Check sheet for the drawn part. Datum: minimum x, y, z corner. Units: mm. Give positions to 0.01 mm unless a question says otherwise; leave off trailing zeros. Order: outer loops, then holes, each group sorted by start corner. A loop starts at its lowest first (then second) coordinate and runs counter-clockwise, first axis right, second up. Notation, with made-up numbers: (72.5, 5) - (120.5, 5) arc R21 ccw to (120.5, 17) - close; hole circle Ø5 at (19, 76.25). An arc over 180 degrees is marked (long way). Answer as a JSON object with one key per item and string values. Group by question number.
(1) Depth check by flat-ended pin: pin 1 Ø5.5 at (y, z) = (11, 181) entering from -X; pin 2 Ø5.5 at (x, y) = (7, 10.5) entering from +Z; pin 3 Ø5.5 at (x, y) = (446.5, 12) entering from +Z; pin 4 Ø2 at (y, z) = (13, 117.5) entering from -X. Enter the tip coordinate at first touch or a pass-through.
(2) Section check A-A (y = 9.25). Record the boundary of the cut face in (x, z), then the cut area to 3 significant figures.
(3) Section check B-B (z = 49.5). Record the boundary of the cut face in (x, y), then the cut area to 3 significant figures.
(4) Thickness scan on line 1 (X direction, y = 10.75, z = 176); line 2 (X direction, y = 5.75, z = 142.5). Record the ranges inside material, lowest first.
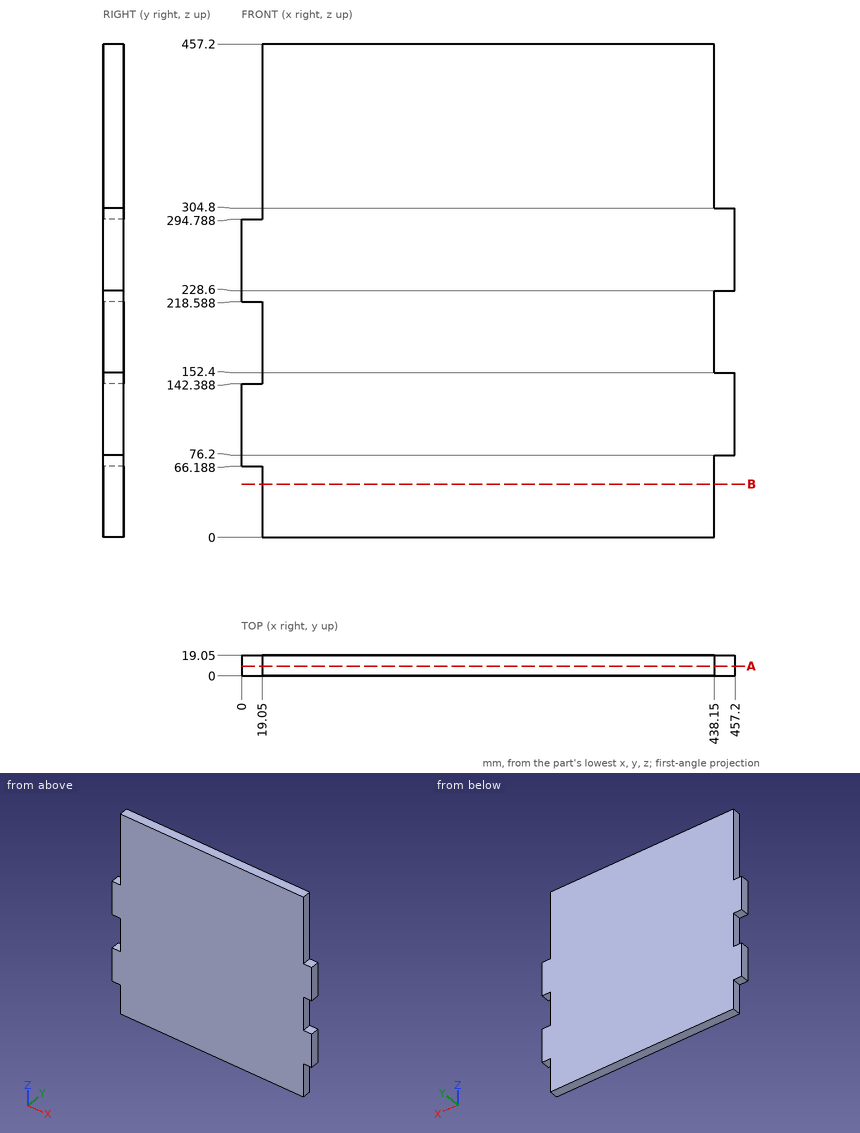
Solutions:
{
 "1": {"pin 1": "stops at x = 19.05", "pin 2": "stops at z = 294.79", "pin 3": "stops at z = 304.8", "pin 4": "stops at x = 0"},
 "2": {"outline": "(0, 66.19) - (19.05, 66.19) - (19.05, 0) - (438.15, 0) - (438.15, 76.2) - (457.2, 76.2) - (457.2, 152.4) - (438.15, 152.4) - (438.15, 228.6) - (457.2, 228.6) - (457.2, 304.8) - (438.15, 304.8) - (438.15, 457.2) - (19.05, 457.2) - (19.05, 294.79) - (0, 294.79) - (0, 218.59) - (19.05, 218.59) - (19.05, 142.39) - (0, 142.39) - close", "area": "197,000 mm2"},
 "3": {"outline": "(19.05, 0) - (438.15, 0) - (438.15, 19.05) - (19.05, 19.05) - close", "area": "7,980 mm2"},
 "4": {"line 1": "x = 19.05 to 438.15", "line 2": "x = 19.05 to 457.2"}
}
